Here's how the part is built. I have some questions about the finished solid (model axes, mm). A direction names the side the tool comes from. Give positions to 0.01 mm unless a question says otherwise; leave off trailing zeros. Write each loop counter-clockwise with the first axis right and the second up, starting at its lowest first coordinate (ties: lowest second). Pieces come first, ordered by that corner, then holes. Notation, with made-up numbers: (70.5, 84.5) -> (76.5, 84.5) arc R17 cw to (76.5, 115.5) -> close; hole circle Ø8 at (39, -4). An arc over 180 degrees is marked (long way). Return JSON: item names as keys, results as strings.
from build123d import *

# Parameters (mm, degrees)
F0_R     = 3.175
F1_DEPTH = 31.75
F2_W     = 12.7
F2_H     = 1.5875
F3_DEPTH = 22.225
F4_W     = 15.875
F4_H     = 6.35
F4_W_2   = 9.525
F5_DEPTH = 25.4


with BuildPart() as f1:
    # F0 (on Front) → F1 (new body)
    with BuildSketch(Plane.XZ):
        with BuildLine():
            Line((15.875, -15.875), (15.875, 0))
            Line((15.875, 0), (-15.875, 0))
            Line((-15.875, 0), (-15.875, -31.75))
            Line((-15.875, -31.75), (0, -31.75))
            ThreePointArc((0, -31.75), (11.22532, -27.10032), (15.875, -15.875))
        make_face()
        with Locations((0, -15.875)):
            Circle(F0_R, mode=Mode.SUBTRACT)
    extrude(amount=-F1_DEPTH)

    # F2 (on face) → F3 (cut)
    with BuildSketch(Plane(origin=(-15.875, 0, 0), x_dir=(0, -1, 0), z_dir=(-1, 0, 0))):
        with Locations((-17.78, -2.38125)):
            Rectangle(F2_W, F2_H)
    extrude(amount=-F3_DEPTH, mode=Mode.SUBTRACT)

    # F4 (on face) → F5 (cut)
    with BuildSketch(Plane(origin=(0, 0, -31.75), x_dir=(1, 0, 0), z_dir=(0, 0, -1))):
        with Locations((7.9375, -15.875)):
            Rectangle(F4_W, F4_H)
        with Locations((-4.7625, -15.875)):
            Rectangle(F4_W_2, F4_H)
    extrude(amount=-F5_DEPTH, mode=Mode.SUBTRACT)


solid = f1.part
1. Suppose I cut it at B-B, the plane z = -14. List the corners of the cut face in (x, y) for me (3 decimals).
Taken from the geometry:
{"outline": "(-15.875, 0) -> (-2.562, 0) -> (-2.562, 12.7) -> (-9.525, 12.7) -> (-9.525, 19.05) -> (-2.562, 19.05) -> (-2.562, 31.75) -> (-15.875, 31.75) -> close; (2.562, 0) -> (15.875, 0) -> (15.875, 12.7) -> (2.562, 12.7) -> close; (2.562, 19.05) -> (15.875, 19.05) -> (15.875, 31.75) -> (2.562, 31.75) -> close"}
2. If I drill on line 1 (Y direction, x = 4.5, z = -19); line 2 (Z direction, x = 0, y = 8.5); line 3 (Y direction, x = -2.5, z = -2.5), over which ranges is the centre line in solid material (lowest first)? Write a range as [from, to].
Taken from the geometry:
{"line 1": "y = [0, 12.7], [19.05, 31.75]", "line 2": "z = [-31.75, -19.05], [-12.7, 0]", "line 3": "y = [0, 11.43], [24.13, 31.75]"}
3. For pin 1 Ø0.5 at (y, z) = (18, -2.5) entering from -X; pin 2 Ø5 at (y, z) = (17, -24) entering from +X; pin 3 Ø6 at (x, y) = (7.5, 24.5) entering from -Z; pin 4 Ø5.5 at (x, z) = (0, -15.875) entering from +Y, each with a flat end and sliding along its axis, tell me the tip position at first contact or that it passes through.
Taken from the geometry:
{"pin 1": "stops at x = 6.35", "pin 2": "stops at x = 14.39", "pin 3": "stops at z = -31.1", "pin 4": "passes through"}
4. If we mould it in two halves opening along X, with no side actions, what happens to faces 1 (the face through (3.03, 25.31, -14.92)), 2 (the face through (-5, 18, -3.175)), 3 (the face through (-15.875, 16, -16)), 4 (the face through (11.101, 6.261, -27.223))? For each: released by +X, released by -X, zero draft, split by the parting line, or undercut.
Taken from the geometry:
{"face 1": "undercut", "face 2": "zero draft", "face 3": "released by -X", "face 4": "released by +X"}
5. Suppose I cut it at A-A, the plane y = 29. List the corners of the cut face in (x, z) for me (3 decimals), and give its area (3 significant figures).
Taken from the geometry:
{"outline": "(-15.875, -31.75) -> (0, -31.75) arc R15.875 ccw to (15.875, -15.875) -> (15.875, 0) -> (-15.875, 0) -> close; hole circle Ø6.35 at (0, -15.875)", "area": "922 mm²"}
6. Which directions (+Z, -Z, +X, -X, +Y, -Y) give clear straight access to the entire face, cutting with the end or side of a thin tool? Please do faces 5 (the face through (-5, 18, -1.588)), 6 (the face through (-10, 16, -31.75)), 7 (the face through (3, 16, -6.35)).
Taken from the geometry:
{"face 5": "-X", "face 6": "-Z, +X, -X, +Y, -Y", "face 7": "-Z, +X"}
